```python
from build123d import *

# Parameters (mm, degrees)
F0_R         = 1.75
F0_R_2       = 17.5
F1_DEPTH     = 2.85
F2_W         = 20
F2_H         = 4
F3_DEPTH     = 14.6
F4_W         = 17
F4_H         = 12.41
F5_DEPTH     = 25
F3_FACE1_W   = 20
F3_FACE1_H   = 17.45
F3_FACE1_W_2 = 17
F3_FACE1_H_2 = 12.41
F9_W         = 20
F9_H         = 17.45
F10_DEPTH    = 1.5
F11_W        = 16.7262982869
F11_H        = 2.3696432114
F12_DEPTH    = 16.4
F13_T1_DEPTH = 20
F13_T3_DEPTH = 31.3016516107
F13_T5_DEPTH = 29.4336950122
F13_T7_DEPTH = 37.8535710714
F4_W_2       = 20
F4_H_2       = 14.6
F14_DEPTH    = 3
F16_DEPTH    = 25


# Not quite as in the source:
# - a fillet or chamfer that OpenCascade refuses, or shapes differently, is made with other operations: its cross-section is extruded or revolved along the edge and cut away or added


with BuildPart() as f1:
    # F0 (on Top) → F1 (new body)
    with BuildSketch(Plane.XY):
        with BuildLine():
            Line((-6.5, -26.5), (19.5, -26.5))
            ThreePointArc((19.5, -26.5), (24.4497474683, -24.4497474683), (26.5, -19.5))
            Line((26.5, -19.5), (26.5, 6.5))
            ThreePointArc((26.5, 6.5), (20.6421356237, 20.6421356237), (6.5, 26.5))
            Line((6.5, 26.5), (-21.5, 26.5))
            ThreePointArc((-21.5, 26.5), (-25.0355339059, 25.0355339059), (-26.5, 21.5))
            Line((-26.5, 21.5), (-26.5, -26.5))
            Line((-26.5, -26.5), (-26.5, -30.5))
            Line((-26.5, -30.5), (-6.5, -30.5))
            Line((-6.5, -30.5), (-6.5, -26.5))
        make_face()
        with Locations((20.6, -19.0101229506)):
            Circle(F0_R, mode=Mode.SUBTRACT)
        with Locations((-19.75, 21.25)):
            Circle(F0_R, mode=Mode.SUBTRACT)
        Circle(F0_R_2, mode=Mode.SUBTRACT)
    extrude(amount=F1_DEPTH)

    # F2 (on face) → F3 (join)
    with BuildSketch(Plane(origin=(0, 0, 0), x_dir=(1, 0, 0), z_dir=(0, 0, -1))):
        with Locations((-16.5, 28.5)):
            Rectangle(F2_W, F2_H)
    extrude(amount=F3_DEPTH)

    # F4 (on face) → F5 (cut)
    with BuildSketch(Plane(origin=(0, -26.5, 0), x_dir=(-1, 0, 0), z_dir=(0, 1, 0))):
        with Locations((16.5, -7.3)):
            Rectangle(F4_W, F4_H)
    extrude(amount=-F5_DEPTH, mode=Mode.SUBTRACT)

    # F8: sweep along a path in F7
    with BuildLine(Plane.YZ.offset(-16.5)) as f8_path:
        Line((-30.5838297752, -0.1396118733), (-52.5838297752, -25.1396118733))
    # F3_face1 (on face) → F8 (sweep)
    with BuildSketch(Plane(origin=(-16.5, -30.5, -3.6969789176), x_dir=(1, 0, 0), z_dir=(0, -1, 0))):
        with Locations((0, -2.1780210824)):
            Rectangle(F3_FACE1_W, F3_FACE1_H)
        with Locations((0, -3.6030210824)):
            Rectangle(F3_FACE1_W_2, F3_FACE1_H_2, mode=Mode.SUBTRACT)
    sweep(path=f8_path.line)

    # F9 (on face) → F10 (join)
    with BuildSketch(Plane.XZ.offset(52.5)):
        with Locations((-16.5, -30.875)):
            Rectangle(F9_W, F9_H)
    extrude(amount=-F10_DEPTH)

    # F11 (on face) → F12 (cut)
    with BuildSketch(Plane(origin=(0, 0, -39.6), x_dir=(1, 0, 0), z_dir=(0, 0, -1))):
        with Locations((-16.5000008565, 49.8151783943)):
            Rectangle(F11_W, F11_H)
    extrude(amount=-F12_DEPTH, mode=Mode.SUBTRACT)

    # F13: fillet of radius 5 on 4 edges, made by hand

    # F13_s2 → F13_t1 (join)
    with BuildSketch(Plane.YZ.offset(-26.5)):
        with BuildLine():
            ThreePointArc((-31.9932372625, -16.2968605255), (-30.299318025, -15.0439217867), (-28.2396696779, -14.6))
            Line((-28.2396696779, -14.6), (-30.5, -14.6))
            Line((-30.5, -14.6), (-31.9932372625, -16.2968605255))
        make_face()
    extrude(amount=F13_T1_DEPTH)

    # F13_s4 → F13_t3 (cut)
    with BuildSketch(Plane.YZ.offset(-32.1508258053)):
        with BuildLine():
            ThreePointArc((-28.2396696779, 2.85), (-30.299318025, 2.4060782133), (-31.9932372625, 1.1531394745))
            Line((-31.9932372625, 1.1531394745), (-30.5, 2.85))
            Line((-30.5, 2.85), (-28.2396696779, 2.85))
        make_face()
    extrude(amount=F13_T3_DEPTH, mode=Mode.SUBTRACT)

    # F13_s6 → F13_t5 (cut)
    with BuildSketch(Plane.YZ.offset(-31.2168475061)):
        with BuildLine():
            ThreePointArc((-52.5, -24.0367390024), (-52.1780251134, -22.2714965153), (-51.2535675846, -20.733599528))
            Line((-51.2535675846, -20.733599528), (-52.5, -22.15))
            Line((-52.5, -22.15), (-52.5, -24.0367390024))
        make_face()
    extrude(amount=F13_T5_DEPTH, mode=Mode.SUBTRACT)

    # F13_s8 → F13_t7 (cut)
    with BuildSketch(Plane.YZ.offset(-35.4267855357)):
        with BuildLine():
            ThreePointArc((-51, -39.6), (-52.1097722286, -37.9657774588), (-52.5, -36.0292857857))
            Line((-52.5, -36.0292857857), (-52.5, -39.6))
            Line((-52.5, -39.6), (-51, -39.6))
        make_face()
    extrude(amount=F13_T7_DEPTH, mode=Mode.SUBTRACT)

    # F4 (on face) → F14 (join)
    with BuildSketch(Plane(origin=(0, -26.5, 0), x_dir=(-1, 0, 0), z_dir=(0, 1, 0))):
        with Locations((16.5, -7.3)):
            Rectangle(F4_W_2, F4_H_2)
        with Locations((16.5, -7.3)):
            Rectangle(F4_W, F4_H, mode=Mode.SUBTRACT)
    extrude(amount=F14_DEPTH)

    # F15 (on face) → F16 (cut)
    with BuildSketch(Plane.XZ.offset(52.5)):
        with BuildLine():
            Line((-12.5835244641, -36.0292857857), (-20.4164755359, -36.0292857857))
            ThreePointArc((-20.4164755359, -36.0292857857), (-16.5, -39.9457613216), (-12.5835244641, -36.0292857857))
        make_face()
    extrude(amount=-F16_DEPTH, mode=Mode.SUBTRACT)


solid = f1.part
```
Build history of the part. All positions in model axes, mm. A direction names the side the tool comes from. Round coordinates to 2 decimals unless told otherwise and drop trailing zeros. Loops run counter-clockwise (first coordinate to the right, second up) from the corner with the lowest first, then second, coordinate; pieces in that order, holes last.
Item 1: Which spindle directions (+Z, -Z, +X, -X, +Y, -Y) get a long thin tool onto all of the face, cutting with end or side? Do faces 1 (the face through (-24.863, -50, -36)), 2 (the face through (-16, -23.5, -14)), 3 (the face through (6, -26.5, 1)), 4 (the face through (-16, -27, -13.505)), 5 (the face through (-8, -37, -16)). Say none if no direction does.
Item 2: Saw through at C-C (z = -27). List the corners of the cut face in (x, y), then the cut area to 3 significant figures.
Item 3: Drill centre lines: line 1 along X through (y, z) = (-29, -7.5); line 2 along Y through (x, z) = (0, 0.7); line 3 along Z through (x, y) = (-19.5, -39.5). Where is each one in solid material? Low to high.
Item 4: Saw through at A-A (x = 0). List the corners of the cut face in (y, z), then the cut area to 3 significant figures.
Item 5: Saw through at B-B (y = -14). List the corners of the cut face in (x, z).
Item 6: Pin check, flat tips, straight feed: P1, Ø1.9, axis at y = -50.5, z = -37, coming from the +X side; P2, Ø10, axis at x = -3, z = -21.5, coming from the -Y side; P3, Ø0.8, axis at x = -15, y = -52, coming from the -Z side; P4, Ø11.5, axis at x = -16.5, z = -7, coming from the +Y side. Stop position of each tip, or through.
Item 7: Saw through at D-D (z = -7.5). List the corners of the cut face in (x, y), then the cut area to 3 significant figures.
Item 8: Two-plate mould, pull along Y, no slides. Class faces 6 (the face through (-19.978, 22.985, 1.405)), 7 (the face through (-16.64, -30.27, 2.42)), 8 (the face through (-26.5, -29, -11)): released by +Y, released by -Y, zero draft, split by the parting line, or undercut.
Worked answers:
1. face 1: -Z
1. face 2: -Z, +X, -X, +Y
1. face 3: +Z, -Z, +X, -Y
1. face 4: +Y
1. face 5: none
2. outline: (-26.5, -52.5) - (-6.5, -52.5) - (-6.5, -41.41) - (-26.5, -41.41) - close; hole (-25, -51) - (-8, -51) - (-8, -42.38) - (-25, -42.38) - close
2. area: 75.1 mm2
3. line 1: x = -26.5 to -25, -8 to -6.5
3. line 2: y = -26.5 to -17.5, 17.5 to 26.5
3. line 3: z = -24.83 to -23.73, -11.32 to -7.38
4. outline: (-26.5, 0) - (-17.5, 0) - (-17.5, 2.85) - (-26.5, 2.85) - close; (17.5, 0) - (26.5, 0) - (26.5, 2.85) - (17.5, 2.85) - close
4. area: 51.3 mm2
5. outline: (-26.5, 0) - (-10.5, 0) - (-10.5, 2.85) - (-26.5, 2.85) - close; (10.5, 0) - (26.5, 0) - (26.5, 2.85) - (10.5, 2.85) - close
6. P1: stops at x = -6.5
6. P2: stops at y = -52.5
6. P3: stops at z = -36.03
6. P4: stops at y = -30.64
7. outline: (-26.5, -39.61) - (-6.5, -39.61) - (-6.5, -23.5) - (-8, -23.5) - (-8, -36.14) - (-25, -36.14) - (-25, -23.5) - (-26.5, -23.5) - close
7. area: 107 mm2
8. face 6: undercut
8. face 7: released by -Y
8. face 8: zero draft
